```python
from build123d import *

# Parameters (mm, degrees)
F1_DEPTH = 6.35
F2_R     = 1.27


with BuildPart() as f1:
    # F0 (on Front) → F1 (new body)
    with BuildSketch(Plane.XZ):
        Polygon((0, 28.9144045194), (-8.8481841409, 5.1053802343), (-33.9983782601, 1.5518276782), (-10.8810784623, -8.9719762946), (-21.404882435, -32.0892760924), (0, -18.4148105473), align=None)
        Polygon((8.8481841409, 5.1053802343), (0, 28.9144045194), (0, -18.4148105473), (21.404882435, -32.0892760924), (10.8810784623, -8.9719762946), (33.9983782601, 1.5518276782), align=None)
    extrude(amount=F1_DEPTH)

    # F2
    f2_edges = [f1.edges().sort_by_distance(p)[0] for p in [
        (-10.702441, 0, -25.252043),
        (-10.702441, -6.35, -25.252043),
        (10.702441, 0, -25.252043),
        (10.702441, -6.35, -25.252043),
        (16.14298, 0, -20.530626),
        (16.14298, -6.35, -20.530626),
        (22.439728, -6.35, -3.710074),
        (22.439728, 0, -3.710074),
        (21.423281, -6.35, 3.328604),
        (21.423281, 0, 3.328604),
        (0, -3.175, 28.914405),
        (-8.848184, -3.175, 5.10538),
        (-4.424092, 0, 17.009892),
        (-4.424092, -6.35, 17.009892),
        (8.848184, -3.175, 5.10538),
        (4.424092, 0, 17.009892),
        (4.424092, -6.35, 17.009892),
        (10.881078, -3.175, -8.971976),
        (33.998378, -3.175, 1.551828),
        (21.404882, -3.175, -32.089276),
        (0, -3.175, -18.414811),
        (-10.881078, -3.175, -8.971976),
        (-21.404882, -3.175, -32.089276),
        (-16.14298, 0, -20.530626),
        (-16.14298, -6.35, -20.530626),
        (-33.998378, -3.175, 1.551828),
        (-21.423281, 0, 3.328604),
        (-21.423281, -6.35, 3.328604),
        (-22.439728, 0, -3.710074),
        (-22.439728, -6.35, -3.710074),
    ]]
    fillet(f2_edges, radius=F2_R)


solid = f1.part
```
Check sheet for the modelled part. Datum: model origin and axes. Units: mm. A direction names the side the tool comes from. Round coordinates to 2 decimals unless told otherwise and drop trailing zeros. Loops run counter-clockwise (first coordinate to the right, second up) from the corner with the lowest first, then second, coordinate; pieces in that order, holes last. Notation, with made-up numbers: (-23.5, 79.25) - (31.5, 79.25) arc R29 ccw to (31.5, 100.25) - close; hole circle Ø4 at (-35, 34). An arc over 180 degrees is marked (long way). Write item = value, one per line. Start each with the question number.
Q1. Section check A-A (y = -3.5). Record the boundary of the cut face in (x, z).
Q2. Thickness scan on L1, parallel to Z at x = 11.5, y = -1.25; L2, parallel to Z at x = -17.5, y = -0.75; L3, parallel to X at y = -0.5, z = -25. Record the ranges inside material, lowest first.
Q3. Release check for a two-part mould opening along Z. For faces 1 (the face through (20.91, -3.148, -4.406)), 2 (the face through (0, 0, -4)), 3 (the face through (-4.836, -3.148, 15.902)) record: pulls with the +Z half, pulls with the -Z half, needs draft (parallel to the pull), parting line crosses it, or undercut.
Q4. Access from +Z, -Z, +X, -X, +Y, -Y to the whole of each face (thin tool, end or side, straight path). Record for faces 4 (the face through (-15.24, -5.97, -19.43)), 5 (the face through (-15.24, -0.38, -19.43)), 6 (the face through (-9.31, -5.97, -23.93)), 7 (the face through (15.13, -5.97, -19.18)), 8 (the face through (21.01, -0.38, -3.96)).
Q5. Depth check by flat-ended pin: P1, Ø10, axis at x = 10.5, z = 14, coming from the -Y side. Enter the tip coordinate at first touch or a pass-through.
Derived:
q1.outline = (-30.04, -0.25) - (-12.04, -8.45) arc R1.27 cw to (-11.41, -10.13) - (-19.63, -28.18) arc R1.27 ccw to (-17.79, -29.78) - (-0.68, -18.85) arc R1.27 cw to (0.68, -18.85) - (17.79, -29.78) arc R1.27 ccw to (19.63, -28.18) - (11.41, -10.13) arc R1.27 cw to (12.04, -8.45) - (30.04, -0.25) arc R1.27 ccw to (29.69, 2.16) - (9.6, 5) arc R1.27 cw to (8.58, 5.81) - (1.19, 25.71) arc R1.27 ccw to (-1.19, 25.71) - (-8.58, 5.81) arc R1.27 cw to (-9.6, 5) - (-29.69, 2.16) arc R1.27 ccw to start
q2.L1 = -25.76 to -10.33, -8.91 to 4.73
q2.L2 = -29.46 to -23.78, -5.84 to 3.77
q2.L3 = -17.89 to -10.79, 10.79 to 17.89
q3.face_1 = undercut
q3.face_2 = needs draft
q3.face_3 = pulls with the +Z half
q4.face_4 = -X, -Y
q4.face_5 = -X, +Y
q4.face_6 = -Z, -Y
q4.face_7 = +X, -Y
q4.face_8 = +X, +Y
q5.P1 = -5.96
